Part model, mm, in its own coordinate system. A direction names the side the tool comes from. Give positions to 0.01 mm unless a question says otherwise; leave off trailing zeros. Write each loop counter-clockwise with the first axis right and the second up, starting at its lowest first coordinate (ties: lowest second). Pieces come first, ordered by that corner, then holes. Notation, with made-up numbers: M 27.25,-10 L 39.25,-10 A27 cw 39.25,10 Z; hole C -14,-23.75 d2. An arc over 180 degrees is marked long. Answer as CSV lines item,"result". Start each with the question number.
1) Slice it at A-A, the plane z = -21. Give the cut face in (x, y).
2) Tool access for faces 4 (the flat face through (0, 14.5, 124)), 5 (the flat face through (0, 3, 195.706)), 6 (the cylindrical face through (10.648, -13.887, 116.677)), 7 (the flat face through (-2, 10, 177)), 8 (the flat face through (8, 13, -74.294)): list every direction of +Z, -Z, +X, -X, +Y, -Y with a clear straight run to the whole face (end or side of a thin tool).
3) Wall check: line 1 along Z through (x, y) = (0, 9.25); line 2 along Z through (x, y) = (0.5, 4); line 3 along X through (y, z) = (0, 190). Give the ranges that are in metal, low to high. Write a range as from..to.
4) Mould opens along Z. For faces 1 (the flat face through (-13, 12, -29.294)), 2 (the flat face through (-2, 11, -104)), 3 (the flat face through (4, -14, 133.206)) say: pulls with the +Z half, pulls with the -Z half, needs draft (parallel to the pull), parting line crosses it, or undercut.
5) Pin check, flat tips, straight feed: pin 1 Ø2.5 at (y, z) = (12, 176) entering from +X; pin 2 Ø1 at (y, z) = (12.5, 177.5) entering from -X; pin 3 Ø6.5 at (x, z) = (0, 173.5) entering from +Y. Stop position of each tip, or through.
Autodesk Inventor part; units mm, degrees
ref_plane "Work Plane2" through (0, 17.5, 0) normal (0, 1, 0) x (-1, 0, 0)
ref_plane "Work Plane3" through (0, 15, 0) normal (0, 1, 0) x (-1, 0, 0)
ref_plane "YZ Plane" through (0, 0, 0) normal (1, 0, 0) x (0, 1, 0)
sketch "Sketch1" plane through (0, 0, 0) normal (1, 0, 0) x (0, 1, 0)
  line L0 (0, 195.7063) -> (0, -134.2937)
  line L1 (0, 195.7063) -> (14, 195.7063)
  line L2 (15, -134.2937) -> (0, -134.2937)
  line L3 (17.5, 100.7063) -> (22.5, 100.7063)
  line L4 (22.5, 100.7063) -> (22.5, -29.2937)
  line L5 (22.5, -29.2937) -> (17.5, -29.2937)
  line L6 (17.5, 100.7063) -> (17.5, 133.2063)
  line L7 (17.5, 133.2063) -> (14, 133.2063)
  line L8 (17.5, -29.2937) -> (17.5, -74.2937)
  line L9 (17.5, -74.2937) -> (15, -74.2937)
  line L10 (14, 195.7063) -> (14, 133.2063)
  line L11 (15, -74.2937) -> (15, -134.2937)
  point P0 (0, 0)
  point P1 (15.75, 133.2063)
  point P2 (20, -29.2937)
  point P3 (7.5, -134.2937)
  point P4 (16.25, -74.2937)
  dimension "d0" = 330
  dimension "d1" = 28
  dimension "d2" = 35
  dimension "d3" = 45
  dimension "d4" = 35
  dimension "d5" = 30
  dimension "d6" = 95
  dimension "d7" = 62.5
  dimension "d8" = 105
  dimension "d9" = 60
revolve "Revolution1" add sketch "Sketch1" angle 360 about axis through (0, 0, 195.7063) along (0, 0, -1)
thread "Thread3"
chamfer "Chamfer2" distance 1 angle 45 1 edges at (0, -17.5, 133.2063)
thread "Thread4"
ref_plane "Work Plane1" through (0, 14, 0) normal (0, 1, 0) x (-1, 0, 0)
ref_plane "Work Plane2" through (0, 17.5, 0) normal (0, 1, 0) x (-1, 0, 0)
sketch "Sketch2" plane through (0, 14, 0) normal (0, 1, 0) x (-1, 0, 0)
  line L0 (-14, 195.7063) -> (14, 195.7063)
  line L1 (14, 195.7063) -> (14, 133.2063)
  line L2 (-14, 195.7063) -> (-14, 133.2063)
  line L3 (0, 185.7063) -> (0, 168.7063) construction
  line L4 (-4, 185.7063) -> (-4, 168.7063)
  line L5 (4, 168.7063) -> (4, 185.7063)
  arc A0 (4, 185.7063) -> (-4, 185.7063) centre (0, 185.7063) ccw
  arc A1 (-4, 168.7063) -> (4, 168.7063) centre (0, 168.7063) ccw
  point P0 (0, 0)
  point P1 (0, 177.2063)
  point P2 (0, 164.7063)
  point P3 (0, 189.7063)
  dimension "d29" = 25
  dimension "d30" = 6
  dimension "d31" = 8
extrude "Extrusion1" cut sketch "Sketch2" against normal blind 4
sketch "Sketch3" plane through (0, 17.5, 0) normal (0, 1, 0) x (-1, 0, 0)
  arc A0 (-4, 118.2063) -> (4, 118.2063) centre (0, 118.2063) ccw
  line L0 (4, 118.2063) -> (4, 133.2938)
  line L1 (-4, 118.2063) -> (-4, 133.2063)
  line L2 (-14, 133.2063) -> (14, 133.2063)
  point P0 (0, 0)
  point P1 (0, 114.2063)
  point P2 (0, 133.2063)
  point P3 (4, 133.2063)
  dimension "d34" = 8
  dimension "d35" = 19
extrude "Extrusion2" cut sketch "Sketch3" against normal blind 3
ref_plane "Work Plane3" through (0, 15, 0) normal (0, 1, 0) x (-1, 0, 0)
sketch "Sketch4" plane through (0, 15, 0) normal (0, 1, 0) x (-1, 0, 0)
  line L0 (0, -95.7937) -> (0, -112.7937) construction
  line L1 (-4, -95.7937) -> (-4, -112.7937)
  line L2 (4, -112.7937) -> (4, -95.7937)
  arc A0 (4, -95.7937) -> (-4, -95.7937) centre (0, -95.7937) ccw
  arc A1 (-4, -112.7937) -> (4, -112.7937) centre (0, -112.7937) ccw
  line L3 (-15, -134.2937) -> (15, -134.2937)
  point P0 (0, 0)
  point P1 (0, -104.2937)
  point P2 (0, -116.7937)
  point P3 (0, -91.7937)
  dimension "d39" = 8
  dimension "d40" = 25
  dimension "d41" = 17.5
extrude "Extrusion3" cut sketch "Sketch4" against normal blind 4
sketch "Sketch11" plane through (0, 11, 0) normal (0, 1, 0) x (1, 0, 0)
  arc A0 (4, 112.7937) -> (-4, 112.7937) centre (0, 112.7937) ccw
  line L0 (4, 112.7937) -> (4, 104.2937)
  line L1 (4, 112.7937) -> (4, 95.7937)
  line L2 (4, 104.2937) -> (0, 104.2937)
  point P0 (0, 0)
  dimension "d100" = 8.5
  dimension "d101" = 4
sketch "Sketch12" plane through (0, 10, 0) normal (0, 1, 0) x (1, 0, 0)
  arc A0 (-4, -185.7063) -> (4, -185.7063) centre (0, -185.7063) ccw
  line L0 (4, -185.7063) -> (4, -177.2063)
  line L1 (4, -177.2063) -> (0, -177.2063)
  point P0 (0, 0)
  dimension "d102" = 8.5
  dimension "d103" = 4
sketch "Sketch5" plane through (0, 0, 195.7063) normal (0, 0, 1) x (1, 0, 0)
  circle A0 centre (0, 0) radius 3
  circle A1 centre (0, -9) radius 2.25
  dimension "d44" = 6
  dimension "d45" = 4.5
  dimension "d46" = 9
hole "Hole1" at (0, -9, 195.7063) direction (0, 0, -1) diameter 4.5 depth 12 tip angle 118
sketch "Sketch6" plane through (0, 0, 195.7063) normal (0, 0, 1) x (1, 0, 0)
  circle A0 centre (0, 0) radius 14
hole "Hole2" at (0, 0, 195.7063) direction (0, 0, -1) diameter 4.2 depth 15 tip angle 118
thread "Thread5"
sketch "Sketch7" plane through (0, 0, -134.2937) normal (0, 0, -1) x (-1, 0, 0)
  circle A0 centre (0, 0) radius 2.5
  circle A1 centre (0, -9) radius 2.25
  circle A2 centre (0, -9) radius 2.25
  dimension "d63" = 5
hole "Hole3" at (0, -9, -134.2937) direction (0, 0, 1) diameter 4.2 depth 12 tip angle 118
sketch "Sketch8" plane through (0, 0, -134.2937) normal (0, 0, -1) x (-1, 0, 0)
  circle A0 centre (0, 0) radius 15
hole "Hole4" at (0, 0, -134.2937) direction (0, 0, 1) diameter 4 depth 15 tip angle 118
sketch "Sketch9" plane through (0, 10, 0) normal (0, 1, 0) x (1, 0, 0)
  line L0 (4, -168.7063) -> (4, -185.7063)
  point P0 (0, 0)
  point P1 (0, -177.2063)
  dimension "d97" = 4
hole "Hole5" at (0, 10, 177.2063) direction (0, -1, 0) diameter 2.5 depth 7 tip angle 118
thread "Thread7"
sketch "Sketch10" plane through (0, 11, 0) normal (0, 1, 0) x (1, 0, 0)
  line L0 (4, 112.7937) -> (4, 95.7937)
  point P0 (0, 0)
  point P1 (0, 104.2937)
  dimension "d89" = 4
hole "Hole6" at (0, 11, -104.2937) direction (0, -1, 0) diameter 2.5 depth 7 tip angle 118
thread "Thread8"
thread "Thread10"
properties part number "Wał"
Found:
1,outline,"C 0,0 d45"
2,face 4,"+Z, +Y"
2,face 5,"+Z, +X, -X, +Y, -Y"
2,face 6,"+Z"
2,face 7,"+Y"
2,face 8,"-Z"
3,line 1,"-134.29..-105.54, -103.04..175.96, 178.46..195.71"
3,line 2,"-134.29..-105.44, -103.15..176.06, 178.35..195.71"
3,line 3,"-14..-2.1, 2.1..14"
4,face 1,"pulls with the -Z half"
4,face 2,"undercut"
4,face 3,"pulls with the +Z half"
5,pin 1,"x = 8.97"
5,pin 2,"x = -7.21"
5,pin 3,"y = 10"
